Here's how the part is built. I have some questions about the finished solid (model axes, mm). A direction names the side the tool comes from. Give positions to 0.01 mm unless a question says otherwise; leave off trailing zeros. Write each loop counter-clockwise with the first axis right and the second up, starting at its lowest first coordinate (ties: lowest second). Pieces come first, ordered by that corner, then holes. Notation, with made-up numbers: (7.25, -38.5) - (52.25, -38.5) arc R9 cw to (52.25, -23.5) - close; hole circle Ø3 at (35.25, 25.5). An arc over 180 degrees is marked (long way). Write each question's results on one line, items separated by ' | '. Start each with the question number.
Item 1: Suppose I cut it at B-B on z = 15. List the corners of the cut face in (x, y) for me, then the cut area to 3 significant figures.
Item 2: Suppose I cut it at A-A on y = 0. List the corners of the cut face in (x, z) for me, then the cut area to 3 significant figures.
Item 3: Which directions (+Z, -Z, +X, -X, +Y, -Y) give clear straight access to the entire face, cutting with the end or side of a thin tool? Please do faces 1 (the cylindrical face through (-8.95, 9.78, 19.52)), 2 (the cylindrical face through (8.95, -9.78, 19.52)), 3 (the cylindrical face through (6.306, -10.502, 11.591)).
Item 4: Suppose I cut it at C-C on x = -18. List the corners of the cut face in (y, z) for me, then the cut area to 3 significant figures.
Item 5: Suppose I cut it at D-D on z = 11.5. List the corners of the cut face in (x, y) for me, then the cut area to 3 significant figures.
Item 6: We'd pull the mould along Y, two halves only. Please class faces 4 (the cylindrical face through (-11.5, 0.2, 12.9)), 5 (the cylindrical face through (6.296, 10.468, 11.591)), 6 (the flat face through (-21, 0, 13)), 7 (the cylindrical face through (8.92, 9.74, 19.52)): +Y half, -Y half, draft (parallel to the pull), parting line (faces both ways), or undercut.
Item 7: Please list where these lines run through material, in increasing order: line 1 along Y through (x, z) = (-18, 19); line 2 along Y through (x, z) = (0, 2.6); line 3 along X through (y, z) = (0.25, 4.75).
Item 8: Will these pins go through, and if not, where does the flat tip stop? P1, Ø6, axis at y = 2.5, z = 11.5, coming from the -X side; P2, Ø1, axis at x = 19.5, z = 11, coming from the +Y side; P3, Ø5, axis at y = -5.5, z = 17, coming from the +X side; P4, Ø8, axis at x = 15, z = 4, coming from the -Y side.
```python
from build123d import *

# Parameters (mm, degrees)
SKETCH_1_W          = 20
SKETCH_1_H          = 22.3606797749979
EXTRUDE_1_DEPTH     = 5
SKETCH_2_R          = 4.05
CUT_EXTRUDE_1_DEPTH = 5
EXTRUDE_2_DEPTH     = 16
EXTRUDE_START       = -8
EXTRUDE_3_DEPTH     = 8
SKETCH_5_R          = 11.5
CUT_EXTRUDE_2_DEPTH = 3
FILLET_2_R          = 2
SKETCH_6_R          = 1.6000000000000016
CUT_EXTRUDE_3_DEPTH = 13
FILLET_3_R          = 1


with BuildPart() as part:
    # 草图1 → 凸台-拉伸1 (new body)
    with BuildSketch(Plane.XY):
        with BuildLine():
            Line((-10, -11.18033988749895), (-10, 11.18033988749895))
            ThreePointArc((-10, 11.180339887498945), (-14.999999999999998, 1.84e-15), (-10.000000000000004, -11.180339887498944))
        make_face()
        Rectangle(SKETCH_1_W, SKETCH_1_H)
        with BuildLine():
            ThreePointArc((14.999999999999998, 0), (13.69306393762915, 6.123724356957945), (9.999999999999998, 11.180339887498947))
            Line((10, 11.18033988749895), (10, -11.18033988749895))
            ThreePointArc((9.999999999999998, -11.180339887498947), (13.69306393762915, -6.123724356957946), (14.999999999999998, -3.67e-15))
        make_face()
    extrude(amount=EXTRUDE_1_DEPTH)

    # 草图2 → 切除-拉伸1 (cut)
    with BuildSketch(Plane(origin=(0, 0, 0), x_dir=(-1, 0, 0), z_dir=(0, 0, -1))):
        Circle(SKETCH_2_R)
    extrude(amount=-CUT_EXTRUDE_1_DEPTH, mode=Mode.SUBTRACT)

    # 草图3 → 凸台-拉伸2 (add)
    with BuildSketch(Plane.XY.offset(5)):
        with BuildLine():
            Line((-10, 11.18033988749895), (-2.6925824035672443, 11.18033988749895))
            ThreePointArc((-2.6925824035672443, 11.18033988749895), (-11.5, 1.41e-15), (-2.6925824035672443, -11.18033988749895))
            Line((-2.6925824035672443, -11.18033988749895), (-10, -11.18033988749895))
            ThreePointArc((-10, -11.18033988749895), (-15.000000000000002, 1.84e-15), (-10, 11.18033988749895))
        make_face()
        with BuildLine():
            Line((2.692582403567243, 11.18033988749895), (10, 11.18033988749895))
            ThreePointArc((10, 11.18033988749895), (15.000000000000002, 0), (10, -11.18033988749895))
            Line((10, -11.18033988749895), (2.6925824035672443, -11.18033988749895))
            ThreePointArc((2.6925824035672443, -11.18033988749895), (11.5, 0), (2.692582403567243, 11.18033988749895))
        make_face()
    extrude(amount=EXTRUDE_2_DEPTH)

    # 草图4 → 凸台-拉伸3 (add)
    with BuildSketch(Plane.XY.offset(21).offset(EXTRUDE_START)):
        with BuildLine():
            Line((10, -11.18033988749895), (25, -11.18033988749895))
            ThreePointArc((25, -11.18033988749895), (27.386127875258307, 0), (25, 11.180339887498949))
            Line((25, 11.180339887498949), (10, 11.18033988749895))
            ThreePointArc((10, 11.18033988749895), (15.000000000000002, 0), (10, -11.18033988749895))
        make_face()
    extrude_3 = extrude(amount=EXTRUDE_3_DEPTH)

    # 镜向1: 凸台-拉伸3 across plane
    add(extrude_3.mirror(Plane(origin=(0, 0, 0), x_dir=(0, 0, 1), z_dir=(1, 0, 0))))

    # 草图5 → 切除-拉伸2 (cut)
    with BuildSketch(Plane.XY.offset(21)):
        with Locations((0, 17)):
            Circle(SKETCH_5_R)
        with Locations((0, -17)):
            Circle(SKETCH_5_R)
    extrude(amount=-CUT_EXTRUDE_2_DEPTH, mode=Mode.SUBTRACT)

    # 圆角2
    fillet_2_edges = [part.edges().sort_by_distance(p)[0] for p in [
        (14.999999999999998, 3.55e-15, 0),
        (-14.999999999999996, 2.22e-15, 0),
    ]]
    fillet(fillet_2_edges, radius=FILLET_2_R)

    # 草图6 → 切除-拉伸3 (cut)
    with BuildSketch(Plane.XY.offset(21)):
        with Locations((18, 0)):
            Circle(SKETCH_6_R)
        with Locations((-18, 0)):
            Circle(SKETCH_6_R)
    extrude(amount=-CUT_EXTRUDE_3_DEPTH, mode=Mode.SUBTRACT)

    # 圆角3
    fillet_3_edges = [part.edges().sort_by_distance(p)[0] for p in [
        (2.6925824035672443, -11.18033988749895, 11.5),
        (2.6925824035672443, 11.18033988749895, 11.5),
        (-2.6925824035672443, 11.18033988749895, 11.5),
        (-2.6925824035672434, -11.18033988749895, 11.5),
    ]]
    fillet(fillet_3_edges, radius=FILLET_3_R)


solid = part.part
```
Checked values:
1) outline: (-25, -11.18) - (-7.25, -11.18) arc R1 ccw to (-6.67, -9.37) arc R11.5 cw to (-6.67, 9.37) arc R1 ccw to (-7.25, 11.18) - (-25, 11.18) arc R27.39 ccw to start; (6.67, -9.37) arc R1 ccw to (7.25, -11.18) - (25, -11.18) arc R27.39 ccw to (25, 11.18) - (7.25, 11.18) arc R1 ccw to (6.67, 9.37) arc R11.5 cw to start; hole circle Ø3.2 at (-18, 0); hole circle Ø3.2 at (18, 0) | area: 750 mm^2
2) outline: (-27.39, 13) - (-19.6, 13) - (-19.6, 21) - (-27.39, 21) - close; (-16.4, 13) - (-15, 13) - (-15, 2) arc R2 ccw to (-13, 0) - (-4.05, 0) - (-4.05, 5) - (-11.5, 5) - (-11.5, 21) - (-16.4, 21) - close; (4.05, 0) - (13, 0) arc R2 ccw to (15, 2) - (15, 13) - (16.4, 13) - (16.4, 21) - (11.5, 21) - (11.5, 5) - (4.05, 5) - close; (19.6, 13) - (27.39, 13) - (27.39, 21) - (19.6, 21) - close | area: 367 mm^2
3) face 1: +Z, +Y | face 2: +Z, -Y | face 3: +Z
4) outline: (-11.18, 13) - (-1.6, 13) - (-1.6, 21) - (-11.18, 21) - close; (1.6, 13) - (11.18, 13) - (11.18, 21) - (1.6, 21) - close | area: 153 mm^2
5) outline: (-10, -11.18) - (-7.25, -11.18) arc R1 ccw to (-6.67, -9.37) arc R11.5 cw to (-6.67, 9.37) arc R1 ccw to (-7.25, 11.18) - (-10, 11.18) arc R15 ccw to start; (6.67, -9.37) arc R1 ccw to (7.25, -11.18) - (10, -11.18) arc R15 ccw to (10, 11.18) - (7.25, 11.18) arc R1 ccw to (6.67, 9.37) arc R11.5 cw to start | area: 179 mm^2
6) face 4: undercut | face 5: undercut | face 6: draft | face 7: +Y half
7) line 1: y = -11.18 to -1.6, 1.6 to 11.18 | line 2: y = -11.18 to -4.05, 4.05 to 11.18 | line 3: x = -15 to -4.04, 4.04 to 15
8) P1: stops at x = -27.39 | P2: passes through | P3: stops at x = 27.22 | P4: stops at y = -10.2
